Study the drawing (mm; zero at the part's minimum x, y, z) and answer. Give positions to 0.01 mm unless a question says otherwise; leave off trailing zeros. Write each loop counter-clockwise with the first axis right and the second up, starting at its lowest first coordinate (ties: lowest second). Pieces come first, ordered by that corner, then holes. Notation, with made-up numbers: (79.25, 31.25) - (95.25, 31.25) arc R23 ccw to (95.25, 59.25) - close; hole circle Ø11 at (46, -14.75). An arc over 180 degrees is marked (long way). Return JSON: item names as keys, results as strings.
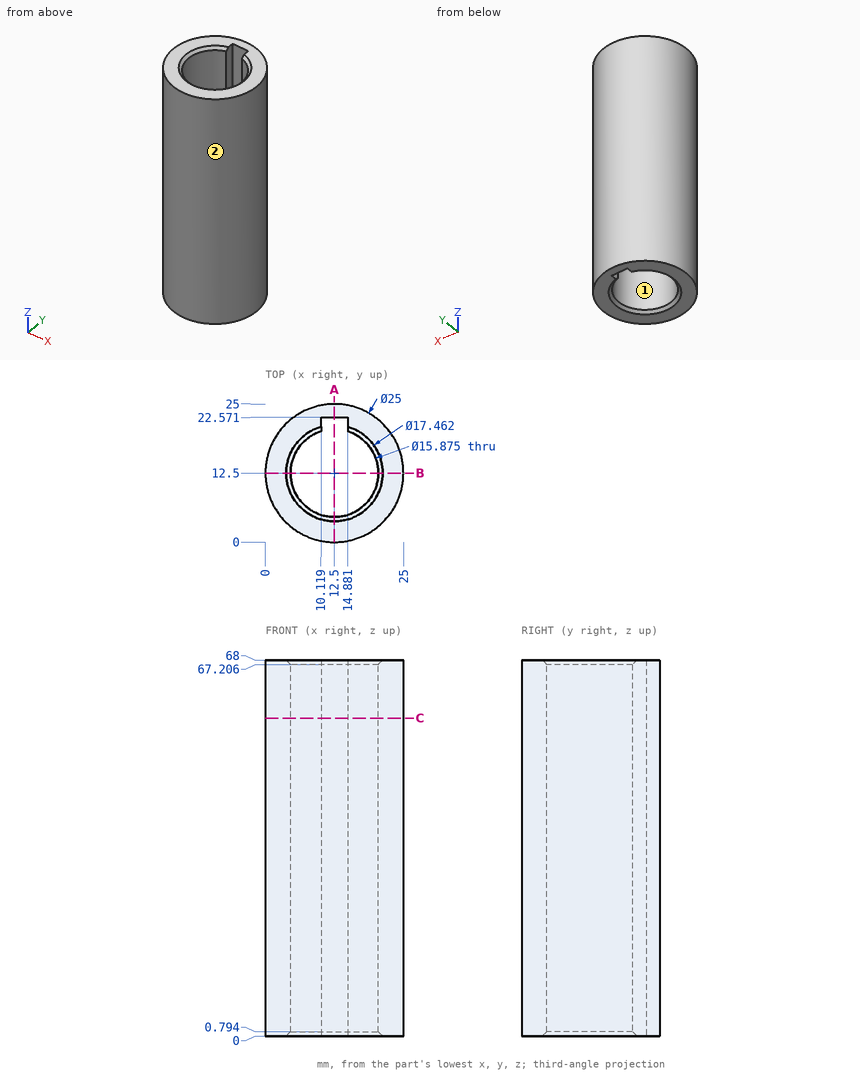
Item 1: A cutting plane is placed at C-C on z = 57.5. Determine the outline of the cut face in (x, y) (1 decimal).
Answer below:
{"outline": "circle Ø25 at (12.5, 12.5); hole (10.1, 20.1) arc R7.9 ccw (long way) to (14.9, 20.1) - (14.9, 22.6) - (10.1, 22.6) - close"}
Item 2: A cutting plane is placed at A-A on x = 12.5. Determine the outline of the cut face in (y, z).
Answer below:
{"outline": "(0, 0) - (3.77, 0) - (4.56, 0.79) - (4.56, 67.21) - (3.77, 68) - (0, 68) - close; (22.57, 0) - (25, 0) - (25, 68) - (22.57, 68) - close"}
Item 3: The mould has two halves that part along X. Classify the marked faces 1 and 2: +X half, -X half, draft (parallel to the pull), parting line (faces both ways), or undercut.
Answer below:
{"face 1": "undercut", "face 2": "parting line"}
Item 4: Flat-ended cylindrical pins translate along their axes: P1, Ø1, axis at x = 16, z = 43, coming from the +Y side (1 decimal); P2, Ø12, axis at x = 6, z = 54, coming from the +Y side; P3, Ø0.7, axis at y = 21.5, z = 47, coming from the -X side (1 decimal); P4, Ø9.5, axis at x = 12.5, y = 12.5, coming from the +Z side. Find the tip coordinate at first contact, or state that the pin passes through.
Answer below:
{"P1": "stops at y = 24.6", "P2": "stops at y = 24.99", "P3": "stops at x = 3.5", "P4": "passes through"}
Item 5: A cutting plane is placed at B-B on y = 12.5. Determine the outline of the cut face in (x, z).
Answer below:
{"outline": "(0, 0) - (3.77, 0) - (4.56, 0.79) - (4.56, 67.21) - (3.77, 68) - (0, 68) - close; (20.44, 0.79) - (21.23, 0) - (25, 0) - (25, 68) - (21.23, 68) - (20.44, 67.21) - close"}
Item 6: Consider L1, parallel to Y at x = 12.5, z = 36; L2, parallel to X at y = 6, z = 35 (1 decimal); L3, parallel to X at y = 18.5, z = 32.5 (1 decimal). Determine where each line is inside the solid, lowest interval first.
Answer below:
{"L1": "y = 0 to 4.56, 22.57 to 25", "L2": "x = 1.8 to 7.9, 17.1 to 23.2", "L3": "x = 1.5 to 7.3, 17.7 to 23.5"}
